Input: part model. Units: mm. Frame: model coordinates. A direction names the side the tool comes from. Give positions to 0.01 mm unless a question says otherwise; leave off trailing zeros. Order: outer loops, then holes, each group sorted by start corner. A loop starts at its lowest first (then second) coordinate and runs counter-clockwise, first axis right, second up. Notation, with made-up numbers: (31.5, 63) -> (84.5, 63) arc R13 ccw to (84.5, 71) -> close; hole circle Ø7 at (86, 34). An arc over 180 degrees is marked (long way). Use a Markdown table: item, result. Add a question column.
from build123d import *

# Parameters (mm, degrees)
SKETCH1_W           = 30
SKETCH1_H           = 23
SKETCH1_R           = 6
SKETCH1_R_2         = 1.5
BOSS_EXTRUDE1_DEPTH = 10
SKETCH2_W           = 2
SKETCH2_H           = 15
CUT_EXTRUDE1_DEPTH  = 10
CUT_EXTRUDE2_REACH  = 41.102
SKETCH3_R           = 2.1
SKETCH4_R           = 1.25
CUT_EXTRUDE3_DEPTH  = 20
FILLET1_R           = 3
FILLET2_R           = 0.5


with BuildPart() as part:
    # Sketch1 → Boss-Extrude1 (new body)
    with BuildSketch(Plane(origin=(0, 0, 0), x_dir=(1, 0, 0), z_dir=(0, 1, 0))):
        with Locations((15, -11.5)):
            Rectangle(SKETCH1_W, SKETCH1_H)
        with Locations(Location((15, -13, 0), (0, 0, 270))):
            Circle(SKETCH1_R, mode=Mode.SUBTRACT)
        with Locations(Location((5, -19.5, 0), (0, 0, 270))):
            Circle(SKETCH1_R_2, mode=Mode.SUBTRACT)
        with Locations(Location((25, -19.5, 0), (0, 0, 270))):
            Circle(SKETCH1_R_2, mode=Mode.SUBTRACT)
    extrude(amount=BOSS_EXTRUDE1_DEPTH)

    # Sketch2 → Cut-Extrude1 (cut)
    with BuildSketch(Plane(origin=(0, 10, 0), x_dir=(1, 0, 0), z_dir=(0, 1, 0))):
        with Locations((15, -4.5)):
            Rectangle(SKETCH2_W, SKETCH2_H)
    extrude(amount=-CUT_EXTRUDE1_DEPTH, mode=Mode.SUBTRACT)

    # Sketch3 → Cut-Extrude2 (cut, up to next)
    with BuildSketch(Plane(origin=(30, 0, 0), x_dir=(0, 0, -1), z_dir=(1, 0, 0)), mode=Mode.PRIVATE) as cut_extrude2_sk1:
        with Locations((-3.5, 5)):
            Circle(SKETCH3_R)
    cut_extrude2_tool1 = extrude(cut_extrude2_sk1.sketch, amount=-CUT_EXTRUDE2_REACH, mode=Mode.PRIVATE) & part.part
    add(cut_extrude2_tool1.solids().sort_by_distance((30, 5, 3.5))[0], mode=Mode.SUBTRACT)

    # Sketch4 → Cut-Extrude3 (cut)
    with BuildSketch(Plane(origin=(14, 0, 0), x_dir=(0, 0, -1), z_dir=(1, 0, 0))):
        with Locations((-3.5, 5)):
            Circle(SKETCH4_R)
    extrude(amount=-CUT_EXTRUDE3_DEPTH, mode=Mode.SUBTRACT)

    # Fillet1
    fillet1_edges = [part.edges().sort_by_distance(p)[0] for p in [
        (30, 5, 23),
        (0, 5, 23),
    ]]
    fillet(fillet1_edges, radius=FILLET1_R)

    # Fillet2
    fillet2_edges = [part.edges().sort_by_distance(p)[0] for p in [
        (14, 5, 7.083920217),
        (16, 5, 7.083920217),
        (16, 5, 0),
        (14, 5, 0),
        (0, 5, 0),
        (30, 5, 0),
    ]]
    fillet(fillet2_edges, radius=FILLET2_R)


solid = part.part
Q1. Section query D-D (z = 19.5). Return loops of the section in (x, y), plus the area to 3 significant figures.
Q2. Section query A-A (x = 5). Return loops of the section in (y, z), plus the area to 3 significant figures.
Q3. Draft query along X for faces 4 (the flat face through (23, 5, 0)), 5 (the flat face through (16, 5, 6)), 6 (the flat face through (30, 5, 10)). Return one class per face: +X half, -X half, draft (parallel to the pull), parting line (faces both ways), or undercut.
Q4. First-contact query: pin 1 (3.5 mm diameter, centred on y = 5, z = 3.5, fed in from +X); pin 2 (2.5 mm diameter, centred on x = 25, z = 19.5, fed in from +Y). Flat tips, straight axial feed; report the tip coordinate or a pass-through.
Q5. Section query C-C (y = 5.75). Return loops of the section in (x, z).
Q6. Ray query, line 1 (X direction, y = 6, z = 5.75); line 2 (Z direction, x = 20.5, y = 3.75); line 3 (X direction, y = 7.5, z = 13). Return the intervals inside material, ascending.
Q7. Access query for faces 1 (the flat face through (14, 6.2, 4.3)), 2 (the cylindrical face through (23.098, 7.082, 3.773)), 3 (the cylindrical face through (26.01, 4.93, 18.39)). Directions: +Z, -Z, +X, -X, +Y, -Y. A direction counts if a zero-diameter tool reaches every point of the face in a straight line with its end or side. Return the directions, or none.
Q8. Section query B-B (z = 13). Return loops of the section in (x, y), plus the area to 3 significant figures.
Solution:
| question | item | result |
|---|---|---|
| 1 | outline | (0, 0) -> (3.5, 0) -> (3.5, 10) -> (0, 10) -> close; (6.5, 0) -> (23.5, 0) -> (23.5, 10) -> (6.5, 10) -> close; (26.5, 0) -> (30, 0) -> (30, 10) -> (26.5, 10) -> close |
| 1 | area | 240 mm² |
| 2 | outline | (0, 0) -> (10, 0) -> (10, 18) -> (0, 18) -> close; (0, 21) -> (10, 21) -> (10, 23) -> (0, 23) -> close; hole circle Ø2.5 at (5, 3.5) |
| 2 | area | 195 mm² |
| 3 | face 4 | draft |
| 3 | face 5 | undercut |
| 3 | face 6 | +X half |
| 4 | pin 1 | stops at x = 14 |
| 4 | pin 2 | passes through |
| 5 | outline | (0, 0.5) arc R0.5 ccw to (0.5, 0) -> (13.5, 0) arc R0.5 ccw to (14, 0.5) -> (14, 2.5) -> (0, 2.5) -> close; (0, 4.5) -> (14, 4.5) -> (14, 6.68) arc R0.5 ccw to (13.62, 7.16) arc R6 cw (long way) to (16.38, 7.16) arc R0.5 ccw to (16, 6.68) -> (16, 5.46) -> (30, 5.46) -> (30, 20) arc R3 ccw to (27, 23) -> (3, 23) arc R3 ccw to (0, 20) -> close; (16, 0.5) arc R0.5 ccw to (16.5, 0) -> (29.5, 0) arc R0.5 ccw to (30, 0.5) -> (30, 1.54) -> (16, 1.54) -> close; hole circle Ø3 at (5, 19.5); hole circle Ø3 at (25, 19.5) |
| 6 | line 1 | x = 0 to 14, 16 to 30 |
| 6 | line 2 | z = 0 to 1.81, 5.19 to 10.6, 15.4 to 23 |
| 6 | line 3 | x = 0 to 9, 21 to 30 |
| 7 | face 1 | -Z, +Y, -Y |
| 7 | face 2 | +X |
| 7 | face 3 | +Y, -Y |
| 8 | outline | (0, 0) -> (9, 0) -> (9, 10) -> (0, 10) -> close; (21, 0) -> (30, 0) -> (30, 10) -> (21, 10) -> close |
| 8 | area | 180 mm² |
